from build123d import *

# Parameters (mm, degrees)
F1_DEPTH = 50
F2_R     = 7.14375
F3_DEPTH = 50.801


with BuildPart() as f1:
    # F0 (on Right) → F1 (new body)
    with BuildSketch(Plane.YZ):
        Polygon((0, -42.8625), (0, 0), (44.45, 0), (44.45, -42.8625), (47.625, -42.8625), (47.625, 3.175), (-3.175, 3.175), (-3.175, -42.8625), align=None)
    extrude(amount=-F1_DEPTH)

    # F2 (on face) → F3 (cut, through all)
    with BuildSketch(Plane(origin=(0, 47.625, 0), x_dir=(-1, 0, 0), z_dir=(0, 1, 0))):
        with Locations((25, -19.84375)):
            Circle(F2_R)
    extrude(amount=-F3_DEPTH, mode=Mode.SUBTRACT)


solid = f1.part
Build history of the part. All positions in model axes, mm. A direction names the side the tool comes from. Give positions to 0.01 mm unless a question says otherwise; leave off trailing zeros. Write each loop counter-clockwise with the first axis right and the second up, starting at its lowest first coordinate (ties: lowest second). Pieces come first, ordered by that corner, then holes. Notation, with made-up numbers: (53, 79) - (93, 79) arc R37 cw to (93, 118) - close; hole circle Ø4 at (-39, 42.25). An arc over 180 degrees is marked (long way). Use one line per item in the form item = value. Start each with the question number.
1. Probe line 1 (Y direction, x = -41.5, z = -33.5) (3 decimals); line 2 (Z direction, x = -25, y = 46.5) (1 decimal); line 3 (Z direction, x = -31.5, y = 44) (3 decimals). List the from-to ranges inside material, lowest first. Write a range as [from, to].
2. Drop flat-ended pins along their axis: pin 1 Ø18.5 at (x, z) = (-25, -19.84) entering from -Y (3 decimals); pin 2 Ø10 at (x, y) = (-44, 37.5) entering from -Z. Give the stop position or say it passes through.
3. Band-saw the part on A-A on z = -9.5. Write the cut outline in (x, y) (3 decimals).
4. 3-axis set-ups, long thin cutter, end or side, ignore diameter. For faces 4 (the face through (-19, 0, -26)), 5 (the face through (-19, 47.625, -25)): which of +Z, -Z, +X, -X, +Y, -Y reach the whole face in a straight line?
5. Band-saw the part on D-D on z = -19. Write the cut outline in (x, y) (3 decimals), plus the area to 3 significant figures.
6. Band-saw the part on B-B on x = -25. Count the separate pieces of the cut face and the enclosed holes in it, plus the area to 3 significant figures.
7. Two-plate mould, pull along Z, no slides. Class faces 1 (the face through (-28.3, -1.57, -26.18)), 2 (the face through (-25, 46, -42.862)), 3 (the face through (-19, -3.175, -14)): released by +Z, released by -Z, zero draft, split by the parting line, or undercut.
Conclusion:
q1.line_1 = [-3.175, 0], [44.45, 47.625]
q1.line_2 = [-42.9, -27], [-12.7, 3.2]
q1.line_3 = [0, 3.175]
q2.pin_1 = -3.175
q2.pin_2 = 0
q3.outline = (-50, -3.175) - (0, -3.175) - (0, 0) - (-50, 0) - close; (-50, 44.45) - (0, 44.45) - (0, 47.625) - (-50, 47.625) - close
q4.face_4 = -Z, +X, -X
q4.face_5 = +Z, -Z, +X, -X, +Y
q5.outline = (-50, -3.175) - (-32.094, -3.175) - (-32.094, 0) - (-50, 0) - close; (-50, 44.45) - (-32.094, 44.45) - (-32.094, 47.625) - (-50, 47.625) - close; (-17.906, -3.175) - (0, -3.175) - (0, 0) - (-17.906, 0) - close; (-17.906, 44.45) - (0, 44.45) - (0, 47.625) - (-17.906, 47.625) - close
q5.area = 227 mm²
q6.separate_pieces = 3
q6.enclosed_holes = 0
q6.area = 343 mm²
q7.face_1 = undercut
q7.face_2 = released by -Z
q7.face_3 = zero draft
